Build history of the part. All positions in model axes, mm. Face numbers are marked on the shaded views. A direction names the side the tool comes from. Give positions to 0.01 mm unless a question says otherwise; leave off trailing zeros. Loops run counter-clockwise (first coordinate to the right, second up) from the corner with the lowest first, then second, coordinate; pieces in that order, holes last. Notation, with made-up numbers: M 42,-30 L 49,-30 A35 ccw 49,3 Z; hole C -35,9 d4. An arc over 180 degrees is marked long. Answer as a JSON object with one key per item and string values. Group by question number.
1. Slice it at B-B (x = 9.25). List the corners of the cut face in (y, z).
2. Drill centre lines: line 1 along Z through (x, y) = (-11, 0.5); line 2 along Z through (x, y) = (3.25, -7); line 3 along Y through (x, z) = (9.5, -70.5). Where is each one in solid material? Low to high. Write a range as [from, to].
3. Slice it at C-C (y = -14). List the corners of the cut face in (x, z).
4. Drop flat-ended pins along their axis: pin 1 Ø11.5 at (x, z) = (-0.5, 10.5) entering from -Y; pin 2 Ø2.5 at (x, z) = (-11.5, 4.5) entering from -Y; pin 3 Ø3 at (x, z) = (12.404, 10.5) entering from -Y. Give the stop position or say it passes through.
5. Slice it at A-A (z = -39.5). List the corners of the cut face in (x, y), then the cut area to 3 significant figures.
6. Mould opens along X. For the marked faces 1, 2, 3 and 4 say: released by +X, released by -X, zero draft, split by the parting line, or undercut.
7. 3-axis set-ups, long thin cutter, end or side, ignore diameter. For the marked faces 5, 6 and 7: which of +Z, -Z, +X, -X, +Y, -Y reach the whole face in a straight line?
Autodesk Inventor part; units mm, degrees
ref_plane "YZ Plane" through (0, 0, 0) normal (1, 0, 0) x (0, 1, 0)
ref_plane "XZ Plane" through (0, 0, 0) normal (0, 1, 0) x (-1, 0, 0)
ref_plane "XY Plane" through (0, 0, 0) normal (0, 0, 1) x (1, 0, 0)
sketch "Sketch1" plane through (0, 0, 0) normal (0, 1, 0) x (-1, 0, 0)
  line L0 (0, 0) -> (0, -62.5)
  line L1 (9.458, 0) -> (9.458, 12.5)
  line L2 (9.458, 12.5) -> (9.458, -12.5)
  line L3 (9.458, 12.5) -> (-14.404, 12.5)
  line L4 (-14.404, 12.5) -> (-14.404, -12.5)
  line L5 (-14.404, -12.5) -> (9.458, -12.5)
  line L6 (-14.404, 12.5) -> (-12.404, 12.5)
  line L7 (-14.404, -12.5) -> (-12.404, -12.5)
  circle A0 centre (0.096, 10.5) radius 1.1
  circle A1 centre (-12.404, 10.5) radius 1.1
  circle A2 centre (-12.404, -10.5) radius 1.1
  circle A3 centre (0.096, -10.5) radius 1.1
  line L8 (9.458, -62.5) -> (9.458, -50)
  line L9 (9.458, -50) -> (9.458, -75)
  line L10 (9.458, -50) -> (-14.404, -50)
  line L11 (-14.404, -50) -> (-14.404, -75)
  line L12 (-14.404, -75) -> (9.458, -75)
  line L13 (-14.404, -50) -> (-12.404, -50)
  line L14 (-14.404, -75) -> (-12.404, -75)
  circle A4 centre (0.096, -52) radius 1.1
  circle A5 centre (-12.404, -52) radius 1.1
  circle A6 centre (-12.404, -73) radius 1.1
  circle A7 centre (0.096, -73) radius 1.1
  line L15 (12.458, 15.5) -> (-17.404, 15.5)
  line L16 (-17.404, 15.5) -> (-17.404, -78)
  line L17 (-17.404, -78) -> (12.458, -78)
  line L18 (12.458, -78) -> (12.458, 15.5)
  line L19 (-14.404, -12.5) -> (-14.404, -50)
  line L20 (9.458, -50) -> (9.458, -12.5)
extrude "Extrusion1" add sketch "Sketch1" against normal blind 3 contours L5 L4 L3 L1 L2 | L5 L20 L10 L0 | L0 L10 L19 L5 | L10 L8 L9 L12 L11 | L18 L17 L16 L15
sketch "Sketch2" plane through (0, 0, 0) normal (0, 1, 0) x (1, 0, 0)
  circle A0 centre (-0.096, -10.5) radius 1.1
  circle A1 centre (-0.096, -10.5) radius 2
  circle A2 centre (12.404, -10.5) radius 1.1
  circle A3 centre (12.404, -10.5) radius 2
  circle A4 centre (12.404, 10.5) radius 1.1
  circle A5 centre (12.404, 10.5) radius 2
  circle A6 centre (-0.096, 10.5) radius 2
  circle A7 centre (-0.096, 52) radius 1.1
  circle A8 centre (-0.096, 52) radius 2
  circle A9 centre (-0.096, 73) radius 1.1
  circle A10 centre (-0.096, 73) radius 2
  circle A11 centre (12.404, 73) radius 1.1
  circle A12 centre (12.404, 73) radius 2
  circle A13 centre (12.404, 52) radius 1.1
  circle A14 centre (12.404, 52) radius 2
  circle A15 centre (-0.096, 73) radius 1.1
  circle A16 centre (12.404, 73) radius 1.1
  circle A17 centre (12.404, 52) radius 1.1
  circle A18 centre (-0.096, 52) radius 1.1
  circle A19 centre (-0.096, 10.5) radius 1.1
  circle A20 centre (12.404, 10.5) radius 1.1
  circle A21 centre (12.404, -10.5) radius 1.1
  circle A22 centre (-0.096, -10.5) radius 1.1
  circle A23 centre (-0.096, 10.5) radius 1.1
  point P0 (0, 0)
  dimension "d21" = 4
  dimension "d22" = 4
  dimension "d23" = 4
  dimension "d24" = 4
  dimension "d25" = 4
  dimension "d26" = 4
  dimension "d27" = 4
  dimension "d28" = 4
extrude "Extrusion2" add sketch "Sketch2" along normal blind 3
extrude "Extrusion3" add sketch "Sketch1" along normal blind 4 contours L18 L17 L16 L15
sketch "Sketch3" plane through (-12.458, -3, -78) normal (-1, 0, 0) x (0, 0, 1)
  line L0 (89.6, 0) -> (87.4, 0)
  line L1 (68.6, 0) -> (66.4, 0)
  line L2 (27.1, 0) -> (24.9, 0)
  line L3 (6.1, 0) -> (3.9, 0)
  line L4 (88.5, 0) -> (88.5, 3)
  line L5 (88.5, 3) -> (88.5, 5)
  line L6 (88.5, 3) -> (88.5, 6)
  line L7 (88.5, 5) -> (67.5, 5)
  line L8 (67.5, 3) -> (67.5, 6)
  line L9 (67.5, 5) -> (67.5, 3)
  line L10 (67.5, 3) -> (88.5, 3)
  line L11 (27.1, 0) -> (24.9, 0)
  line L12 (26, 0) -> (26, 5)
  line L13 (26, 5) -> (5, 5)
  line L14 (5, 3) -> (5, 6)
  line L15 (5, 5) -> (5, 3)
  line L16 (26, 3) -> (5, 3)
  line L17 (5, 3) -> (26, 3)
  dimension "d33" = 2
  dimension "d34" = 5
extrude "Extrusion4" cut sketch "Sketch3" against normal up to surface (3 mm away)
sketch "Sketch4" plane through (-12.458, -3, -78) normal (-1, 0, 0) x (0, 0, 1)
  line L0 (0, 0) -> (93.5, 0)
  line L1 (78, 0) -> (78, -30)
  line L2 (78, -30) -> (83, -30)
  line L3 (83, -30) -> (73, -30)
  line L4 (73, -30) -> (73, 0)
  line L5 (83, -30) -> (83, 0)
  line L6 (73, 0) -> (83, 0)
  line L7 (78, 3) -> (78, -30)
  point P0 (78, -30)
  point P1 (83, 0)
  point P2 (73, 0)
  dimension "d37" = 30
  dimension "d38" = 5
  dimension "d39" = 10
extrude "Extrusion5" add sketch "Sketch4" against normal up to surface (29.862 mm away)
sketch "Sketch5" plane through (-12.458, -33, 5) normal (0, 0, 1) x (1, 0, 0)
  line L0 (0, 0) -> (29.862, 0)
  line L1 (0, 30) -> (0, 0)
  circle A0 centre (14.931, 15) radius 15
  line L2 (29.862, 30) -> (29.862, 0)
  line L3 (29.862, 0) -> (29.862, 15)
  point P0 (12.458, 33)
  point P1 (29.862, 13.5629)
  point P2 (14.931, 0)
  point P3 (0, 13.5629)
extrude "Extrusion6" cut sketch "Sketch5" against normal up to surface (10 mm away) contours L1 A0 L0 | A0 L2 L0
sketch "Sketch6" plane through (-12.458, -3, 5) normal (0, 0, 1) x (1, 0, 0)
  line L0 (29.862, -30) -> (29.862, 0)
  line L1 (29.862, -16.4371) -> (26.862, -16.4371)
  circle A0 centre (26.862, -16.4371) radius 1.1
  arc A1 (0, -16.4371) -> (29.862, -16.4371) centre (14.931, -15) ccw
  circle A2 centre (14.931, -15) radius 4.093
  circle A3 centre (25.9738, -19.7402) radius 1.1
  circle A4 centre (24.191, -22.6593) radius 1.1
  circle A5 centre (21.6581, -24.9579) radius 1.1
  circle A6 centre (18.5801, -26.4498) radius 1.1
  circle A7 centre (15.2065, -27.0141) radius 1.1
  circle A8 centre (11.8106, -26.605) radius 1.1
  circle A9 centre (8.6675, -25.2558) radius 1.1
  circle A10 centre (6.0318, -23.0758) radius 1.1
  circle A11 centre (4.1171, -20.2414) radius 1.1
  circle A12 centre (3.0784, -16.9825) radius 1.1
  circle A13 centre (3, -13.5629) radius 1.1
  point P0 (12.458, 3)
  dimension "d46" = 3
  dimension "d47" = 2.2
  dimension "d50" = 180
extrude "Extrusion7" cut sketch "Sketch6" against normal up to surface (10 mm away) contours A0 | A3 | A4 | A5 | A6 | A7 | A8 | A9 | A10 | A11 | A12 | A13
sketch "Sketch7" plane through (-12.458, -3, 5) normal (0, 0, 1) x (1, 0, 0)
  arc A0 (0, -16.4371) -> (29.862, -16.4371) centre (14.931, -15) ccw
  circle A1 centre (14.931, -15) radius 2
  point P0 (12.458, 3)
  dimension "d54" = 4
extrude "Extrusion8" cut sketch "Sketch7" against normal up to surface (10 mm away)
properties part number "pi_cam_stereo_board"
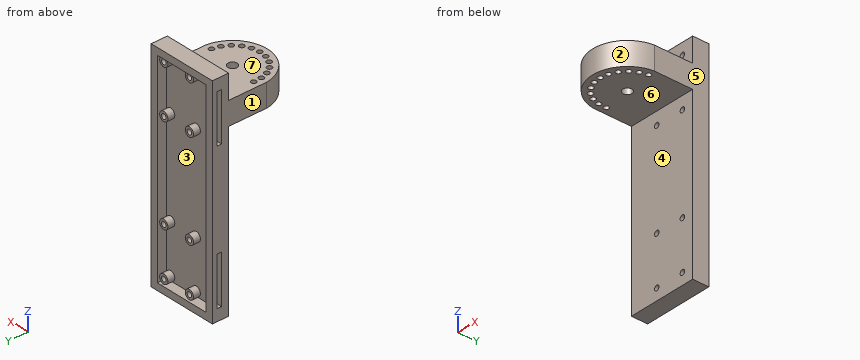
Established:
{
 "1": {"outline": "M -31.38,-5 L -29.06,-5 L -29.06,5 L -31.38,5 Z; M -26.86,-5 L -3,-5 L -3,-78 L 4,-78 L 4,-75 L 0,-75 L 0,12.5 L 4,12.5 L 4,15.5 L -3,15.5 L -3,5 L -26.86,5 Z"},
 "2": {"line 1": "z = [-78, -73], [-52, -10.5], [10.5, 15.5]", "line 2": "z = [-5, 5]", "line 3": "y = [-3, 0]"},
 "3": {"outline": "M -12.46,-5 L 17.4,-5 L 17.4,5 L -12.46,5 Z"},
 "4": {"pin 1": "stops at y = -32.94", "pin 2": "stops at y = -25.95", "pin 3": "stops at y = -3"},
 "5": {"outline": "M -12.46,-3 L 17.4,-3 L 17.4,4 L 14.4,4 L 14.4,0 L -9.46,0 L -9.46,4 L -12.46,4 Z", "area": "114 mm^2"},
 "6": {"face 1": "released by -X", "face 2": "split by the parting line", "face 3": "undercut", "face 4": "zero draft"},
 "7": {"face 5": "+Z, -Z, +X, +Y, -Y", "face 6": "-Z, +X, -X, -Y", "face 7": "+Z, +X, -X, -Y"}
}
